Input: part model. Units: mm. Frame: model coordinates. A direction names the side the tool comes from. Round coordinates to 2 decimals unless told otherwise and drop trailing zeros. Order: outer loops, then holes, each group sorted by start corner. A loop starts at its lowest first (then second) coordinate and runs counter-clockwise, first axis right, second up. Notation, with made-up numbers: (-27.75, 10.25) - (28.25, 10.25) arc R7 cw to (28.25, 15.25) - close; hole circle Ø6 at (66.25, -25). An arc over 180 degrees is marked (long way). One line per item, written item: value. Start each with the question number.
from build123d import *

# Parameters (mm, degrees)
EXTRUDE_1_DEPTH          = 24
SKETCH_3_W               = 8
SKETCH_3_H               = 5
SKETCH_3_H_2             = 6
EXTRUDE_2_DEPTH          = 5
SKETCH_3_4_W             = 8
SKETCH_3_4_H             = 6
EXTRUDE_3_DEPTH          = 85
SKETCH_3_5_W             = 8
SKETCH_3_5_H             = 5
EXTRUDE_5_DEPTH          = 30
SKETCH_4_R               = 15.8
SKETCH_4_R_2             = 9.8
EXTRUDE_4_DEPTH          = 30
FILLET_1_R               = 10
FILLET_2_R               = 4.5
FILLET_3_R               = 20
FILLET_4_R               = 8
FILLET_5_R               = 2
CUT_EXTRUDE_1_DEPTH      = 414.364246156
CUT_EXTRUDE_1_DEPTH_BACK = 414.364246156
SKETCH_5_R               = 2.2
SKETCH_7_R               = 2.2
CUT_EXTRUDE_2_DEPTH      = 10
SKETCH_8_R               = 2.2
CUT_EXTRUDE_3_DEPTH      = 10


with BuildPart() as part:
    # Эскиз1 → Бобышка-Вытянуть1 (new body)
    with BuildSketch(Plane.XY):
        with BuildLine():
            Line((-62, -308), (-94, -308))
            Line((-94, -308), (-100, -308))
            Line((-100, -308), (-100, -302))
            Line((-100, -302), (-94, -302))
            Line((-94, -302), (-94, -293.5))
            Line((-94, -293.5), (-89, -293.5))
            Line((-89, -293.5), (-89, -300))
            Line((-89, -300), (-62, -300))
            ThreePointArc((-62, -300), (-25.937554159, -314.937554159), (-11, -351))
            Line((-11, -351), (-11, -379))
            Line((-11, -379), (-19, -379))
            Line((-19, -379), (-19, -351))
            ThreePointArc((-19, -351), (-31.594408409, -320.594408409), (-62, -308))
        make_face()
    extrude(amount=EXTRUDE_1_DEPTH)

    # Эскиз3 → Бобышка-Вытянуть2 (add)
    with BuildSketch(Plane.XY.offset(24)):
        with BuildLine():
            Line((-19, -351), (-19, -373))
            Line((-19, -373), (-11, -373))
            Line((-11, -373), (-11, -351))
            ThreePointArc((-11, -351), (-25.937554159, -314.937554159), (-62, -300))
            Line((-62, -300), (-89, -300))
            Line((-89, -300), (-89, -308))
            Line((-89, -308), (-62, -308))
            ThreePointArc((-62, -308), (-31.594408409, -320.594408409), (-19, -351))
        make_face()
        with BuildLine():
            Line((-24, -373), (-19, -373))
            Line((-19, -373), (-19, -351))
            ThreePointArc((-19, -351), (-31.594408409, -320.594408409), (-62, -308))
            Line((-62, -308), (-89, -308))
            Line((-89, -308), (-89, -317.132562387))
            Line((-89, -317.132562387), (-70.846385997, -355.21680623))
            ThreePointArc((-70.846385997, -355.21680623), (-64.161644886, -341.441376072), (-52.2, -351))
            ThreePointArc((-52.2, -351), (-57.209156829, -359.549141578), (-67.115881983, -359.358693172))
            Line((-67.115881983, -359.358693172), (-33.582731203, -379.882432752))
            Line((-33.582731203, -379.882432752), (-24, -379.882432752))
            Line((-24, -379.882432752), (-24, -373))
        make_face()
        with BuildLine():
            Line((-19, -385), (-19, -379))
            Line((-19, -379), (-19, -373))
            Line((-19, -373), (-24, -373))
            Line((-24, -373), (-24, -379.882432752))
            Line((-24, -379.882432752), (-33.582731203, -379.882432752))
            Line((-33.582731203, -379.882432752), (-67.115881983, -359.358693172))
            ThreePointArc((-67.115881983, -359.358693172), (-69.281829347, -357.558579218), (-70.846385997, -355.21680623))
            Line((-70.846385997, -355.21680623), (-89, -317.132562387))
            Line((-89, -317.132562387), (-89, -308))
            Line((-89, -308), (-100, -308))
            Line((-100, -308), (-76.26254069, -357.79852433))
            ThreePointArc((-76.26254069, -357.79852433), (-73.740092213, -361.574035882), (-70.248054625, -364.47626042))
            Line((-70.248054625, -364.47626042), (-36.714903846, -385))
            Line((-36.714903846, -385), (-28.714903846, -385))
            Line((-28.714903846, -385), (-19, -385))
        make_face()
        with Locations((-32.714903846, -387.5)):
            Rectangle(SKETCH_3_W, SKETCH_3_H)
        Polygon((-100, -308), (-89, -308), (-89, -300), (-89, -293.5), (-94, -293.5), (-94, -302), (-100, -302), align=None)
        with Locations((-15, -376)):
            Rectangle(SKETCH_3_W, SKETCH_3_H_2)
    extrude(amount=EXTRUDE_2_DEPTH)

    # Эскиз3<4> → Бобышка-Вытянуть3 (add)
    with BuildSketch(Plane.XY.offset(24)):
        with BuildLine():
            Line((-19, -385), (-19, -379))
            Line((-19, -379), (-19, -373))
            Line((-19, -373), (-24, -373))
            Line((-24, -373), (-24, -379.882432752))
            Line((-24, -379.882432752), (-33.582731203, -379.882432752))
            Line((-33.582731203, -379.882432752), (-67.115881983, -359.358693172))
            ThreePointArc((-67.115881983, -359.358693172), (-69.281829347, -357.558579218), (-70.846385997, -355.21680623))
            Line((-70.846385997, -355.21680623), (-89, -317.132562387))
            Line((-89, -317.132562387), (-89, -308))
            Line((-89, -308), (-100, -308))
            Line((-100, -308), (-76.26254069, -357.79852433))
            ThreePointArc((-76.26254069, -357.79852433), (-73.740092213, -361.574035882), (-70.248054625, -364.47626042))
            Line((-70.248054625, -364.47626042), (-36.714903846, -385))
            Line((-36.714903846, -385), (-28.714903846, -385))
            Line((-28.714903846, -385), (-19, -385))
        make_face()
        Polygon((-100, -308), (-89, -308), (-89, -300), (-89, -293.5), (-94, -293.5), (-94, -302), (-100, -302), align=None)
        with Locations((-15, -376)):
            Rectangle(SKETCH_3_4_W, SKETCH_3_4_H)
    extrude(amount=EXTRUDE_3_DEPTH)

    # Эскиз3<5> → Бобышка-Вытянуть5 (add)
    with BuildSketch(Plane.XY.offset(24)):
        with Locations((-32.714903846, -387.5)):
            Rectangle(SKETCH_3_5_W, SKETCH_3_5_H)
    extrude(amount=EXTRUDE_5_DEPTH)

    # Эскиз4 → Бобышка-Вытянуть4 (add)
    with BuildSketch(Plane(origin=(0, 0, 24), x_dir=(-1, 0, 0), z_dir=(0, 0, -1))):
        with Locations((62, -351)):
            Circle(SKETCH_4_R)
        with Locations(Location((62, -351, 0), (0, 0, 334.514265995))):
            Circle(SKETCH_4_R_2, mode=Mode.SUBTRACT)
    extrude(amount=-EXTRUDE_4_DEPTH)

    # Скругление1
    fillet_1_edges = [part.edges().sort_by_distance(p)[0] for p in [
        (-89, -317.132562387, 69),
        (-56.545080529, -365.828481162, 41.5),
        (-76.179159974, -344.029245204, 41.5),
    ]]
    fillet(fillet_1_edges, radius=FILLET_1_R)

    # Скругление2
    fillet_2_edges = [part.edges().sort_by_distance(p)[0] for p in [
        (-36.714903846, -385, 39),
        (-28.714903846, -385, 39),
    ]]
    fillet(fillet_2_edges, radius=FILLET_2_R)

    # Скругление3
    # the kernel refuses this fillet: 20 mm, written as the material it takes off along each edge
    with BuildSketch(Plane(origin=(-100, -308, -3.137524006), x_dir=(0, 1, 0), z_dir=(0, 0, 1))) as fillet_3_piece_1:
        with BuildLine():
            CenterArc((FILLET_3_R * 0.226146033386, -FILLET_3_R), FILLET_3_R, 90, 25.485734005)
            Line((-FILLET_3_R * 0.204140316645, -FILLET_3_R * 0.0973075512795), (-FILLET_3_R * 0.212746043646, -FILLET_3_R * 0.0792537023051))
            Line((-FILLET_3_R * 0.212746043646, -FILLET_3_R * 0.0792537023051), (-FILLET_3_R * 0.00452292066771, FILLET_3_R * 0.02))
            Line((-FILLET_3_R * 0.00452292066771, FILLET_3_R * 0.02), (FILLET_3_R * 0.226146033386, FILLET_3_R * 0.02))
            Line((FILLET_3_R * 0.226146033386, FILLET_3_R * 0.02), (FILLET_3_R * 0.226146033386, 0))
        make_face()
    extrude(amount=139.275048013, mode=Mode.SUBTRACT)

    # Скругление4
    fillet_4_edges = [part.edges().sort_by_distance(p)[0] for p in [
        (-36.714903846, -385, 81.5),
    ]]
    fillet(fillet_4_edges, radius=FILLET_4_R)

    # Скругление5
    fillet_5_edges = [part.edges().sort_by_distance(p)[0] for p in [
        (-99.481868202, -308, 12),
    ]]
    fillet(fillet_5_edges, radius=FILLET_5_R)

    # Эскиз5 → Вырез-Вытянуть1 (cut, two sides: drawn at the far end of the back side and taken through both)
    with BuildSketch(Plane.ZY.offset(94).offset(-CUT_EXTRUDE_1_DEPTH_BACK)):
        with Locations((89.2, -297.75)):
            Circle(SKETCH_5_R)
        with Locations((10, -297.75)):
            Circle(SKETCH_5_R)
        with Locations((49.6, -297.75)):
            Circle(SKETCH_5_R)
    extrude(amount=CUT_EXTRUDE_1_DEPTH + CUT_EXTRUDE_1_DEPTH_BACK, mode=Mode.SUBTRACT)

    # Эскиз7 → Вырез-Вытянуть2 (cut)
    with BuildSketch(Plane.XZ.offset(379)):
        with Locations(Location((-15, 88.8, 0), (0, 0, 270))):
            Circle(SKETCH_7_R)
        with Locations(Location((-15, 48.4, 0), (0, 0, 270))):
            Circle(SKETCH_7_R)
        with Locations(Location((-15, 8, 0), (0, 0, 270))):
            Circle(SKETCH_7_R)
    extrude(amount=-CUT_EXTRUDE_2_DEPTH, mode=Mode.SUBTRACT)

    # Эскиз8 → Вырез-Вытянуть3 (cut)
    with BuildSketch(Plane(origin=(0, 0, 0), x_dir=(-1, 0, 0), z_dir=(0, 0, -1))):
        with Locations((62, -304)):
            Circle(SKETCH_8_R)
        with Locations((28.765981284, -317.765981284)):
            Circle(SKETCH_8_R)
        with Locations((15, -351)):
            Circle(SKETCH_8_R)
    extrude(amount=-CUT_EXTRUDE_3_DEPTH, mode=Mode.SUBTRACT)

    # Зеркальное отражение1: part across plane


with BuildPart() as part_1:
    add(part.part)
    add(part.part.mirror(Plane(origin=(0, 0, 109), x_dir=(1, 0, 0), z_dir=(0, 0, -1))))


solid = part_1.part
1. Section C-C (z = 153.5). Return the cut outline in (x, y).
2. Section D-D (x = -79). Return the cut outline in (y, z), then the cut area to 3 significant figures.
3. Line query: line 1 (X direction, y = -375.15, z = 169.6); line 2 (Z direction, x = -37.5, y = -326.5); line 3 (Y direction, x = -62, z = 7). Output: solid intervals per line, ascending. Write a range as from..to.
4. Pull-direction query (Z, two-part tool) for faces 1 (the face through (-91.465, -299.898, 49.123)), 2 (the face through (-15, -379, 111)), 3 (the face through (-51, -338, 24)); classes: released by +Z, released by -Z, zero draft, split by the parting line, or undercut.
5. Set-up query: faces 4 (the face through (-97, -302, 111)), 5 (the face through (-36.6, -384.71, 108.23)), 6 (the face through (-17, -373, 110)). Return all of +Z, -Z, +X, -X, +Y, -Y with unobstructed straight access to the full face (end or side cutting, diameter ignored); none if empty.
6. Section A-A (y = -297.75). Return the cut outline in (x, z).
7. Section B-B (z = 26.5). Return the cut outline in (x, y).
8. Pin query (flat end, axial travel): pin 1 (3.5 mm diameter, centred on x = -15, y = -351, fed in from -Z); pin 2 (5 mm diameter, centred on x = -46, z = 90, fed in from -Y); pin 3 (5 mm diameter, centred on y = -335, z = 45.5, fed in from -X). Return the tip coordinate at first contact, or that it passes through.
Solved:
1. outline: (-100, -303.48) arc R20 ccw to (-98.05, -312.08) - (-76.26, -357.8) arc R15.8 ccw to (-70.25, -364.48) - (-38.64, -383.82) arc R8 ccw to (-34.46, -385) - (-19, -385) - (-19, -379) - (-11, -379) - (-11, -373) - (-24, -373) - (-24, -379.88) - (-33.58, -379.88) - (-67.12, -359.36) arc R9.8 cw to (-70.85, -355.22) - (-88.03, -319.17) arc R10 cw to (-89, -314.87) - (-89, -293.5) - (-94, -293.5) - (-94, -302) - (-100, -302) - close
2. outline: (-352.06, 24) - (-308, 24) - (-308, 0) - (-300, 0) - (-300, 29) - (-335.56, 29) - (-335.56, 54) - (-338.11, 54) - (-338.11, 164) - (-335.56, 164) - (-335.56, 189) - (-300, 189) - (-300, 218) - (-308, 218) - (-308, 194) - (-352.06, 194) - close
2. area: 3,260 mm²
3. line 1: x = -52.81..-41.31, -24..-17.2, -12.8..-11
3. line 2: z = 24..29, 189..194
3. line 3: y = -308..-306.2, -301.8..-300
4. face 1: undercut
4. face 2: zero draft
4. face 3: released by -Z
5. face 4: +Z, -Z, -X, +Y
5. face 5: -X, -Y
5. face 6: +X, +Y
6. outline: (-94, 0) - (-89, 0) - (-89, 7.8) - (-94, 7.8) - close; (-94, 12.2) - (-89, 12.2) - (-89, 47.4) - (-94, 47.4) - close; (-94, 51.8) - (-89, 51.8) - (-89, 87) - (-94, 87) - close; (-94, 91.4) - (-89, 91.4) - (-89, 126.6) - (-94, 126.6) - close; (-94, 131) - (-89, 131) - (-89, 166.2) - (-94, 166.2) - close; (-94, 170.6) - (-89, 170.6) - (-89, 205.8) - (-94, 205.8) - close; (-94, 210.2) - (-89, 210.2) - (-89, 218) - (-94, 218) - close
7. outline: (-100, -303.48) arc R20 ccw to (-98.05, -312.08) - (-76.26, -357.8) arc R15.8 ccw to (-70.25, -364.48) - (-38.87, -383.68) arc R4.5 cw to (-36.71, -387.52) - (-36.71, -390) - (-28.71, -390) - (-28.71, -389.5) arc R4.5 cw to (-24.21, -385) - (-19, -385) - (-19, -379) - (-11, -379) - (-11, -351) arc R51 ccw to (-62, -300) - (-89, -300) - (-89, -293.5) - (-94, -293.5) - (-94, -302) - (-100, -302) - close; hole circle Ø19.6 at (-62, -351)
8. pin 1: stops at z = 10
8. pin 2: stops at y = -380.85
8. pin 3: stops at x = -88.32
